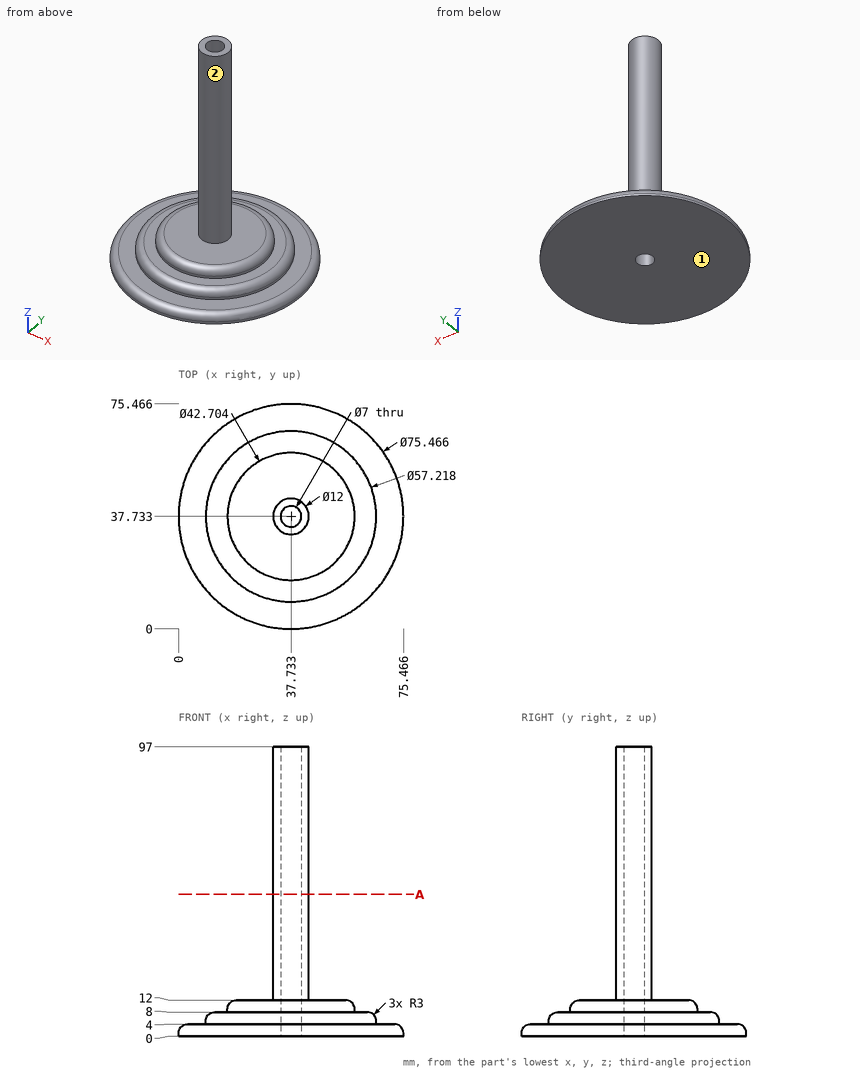
Check sheet for the drawn part. Datum: minimum x, y, z corner. Units: mm. A direction names the side the tool comes from. Round coordinates to 2 decimals unless told otherwise and drop trailing zeros. Order: outer loops, then holes, each group sorted by start corner. A loop starts at its lowest first (then second) coordinate and runs counter-clockwise, first axis right, second up.
1. Access from +Z, -Z, +X, -X, +Y, -Y to the whole of each face (thin tool, end or side, straight path). Record for the marked faces 1 and 2.
Final values:
face 1: -Z, +X, -X, +Y, -Y
face 2: +Z
2. Thickness scan on L1, parallel to Z at x = 67.5, y = 53; L2, parallel to Z at x = 17, y = 29; L3, parallel to X at y = 35, z = 77.5 (1 decimal). Record the ranges inside material, lowest first.
Final values:
L1: z = 0 to 4
L2: z = 0 to 8
L3: x = 32.4 to 35.5, 39.9 to 43.1
3. Go/stop test with flat-tipped pins: P1, Ø6, axis at x = 68, y = 9.5, coming from the -Z side; P2, Ø2, axis at x = 26.5, y = 61, coming from the +Z side; P3, Ø6, axis at x = 37, z = 51.5, coming from the +Y side; P4, Ø12, axis at x = 46.5, z = 73.5, coming from the -Y side. Record where each tip stops, or that it passes through.
Final values:
P1: passes through
P2: stops at z = 8
P3: stops at y = 43.73
P4: stops at y = 32.41
4. Section check A-A on z = 47.5. Record the cut outline in (x, y), then the cut area to 3 significant figures.
Final values:
outline: circle Ø12 at (37.73, 37.73); hole circle Ø7 at (37.73, 37.73)
area: 74.6 mm2
